```python
from build123d import *

# Parameters (mm, degrees)
SKETCH1_W                            = 127
SKETCH1_H                            = 50.8
BOSS_EXTRUDE1_DEPTH                  = 25.4
SKETCH2_R                            = 4.5085
CUT_EXTRUDE1_DEPTH                   = 73.955945611
SKETCH3_W                            = 19.05
SKETCH3_H                            = 1.5875
CUT_EXTRUDE2_DEPTH                   = 73.955945611
SKETCH4_W                            = 12.7
SKETCH4_H                            = 14.605
CUT_EXTRUDE3_DEPTH                   = 73.955945611
F_11_64_0_17188_DIAMETER_HOLE1_D     = 4.365752
F_11_64_0_17188_DIAMETER_HOLE1_DEPTH = 25.4
F_11_64_0_17188_DIAMETER_HOLE1_TIP   = 1.311604225
FILLET3_R                            = 2.54
F_11_64_0_17188_DIAMETER_HOLE2_D     = 4.365752
F_11_64_0_17188_DIAMETER_HOLE2_DEPTH = 25.4
F_11_64_0_17188_DIAMETER_HOLE2_TIP   = 1.311604225
SKETCH9_W                            = 44.45
SKETCH9_H                            = 6.35
CUT_EXTRUDE4_DEPTH                   = 73.955945611


with BuildPart() as part:
    # Sketch1 → Boss-Extrude1 (new body)
    with BuildSketch(Plane(origin=(0, 0, 0), x_dir=(1, 0, 0), z_dir=(0, 1, 0))):
        Rectangle(SKETCH1_W, SKETCH1_H)
    extrude(amount=BOSS_EXTRUDE1_DEPTH)

    # Sketch2 → Cut-Extrude1 (cut, through all)
    with BuildSketch(Plane(origin=(0, 25.4, 0), x_dir=(1, 0, 0), z_dir=(0, 1, 0))):
        with Locations(Location((-44.45, 0, 0), (0, 0, 270))):
            Circle(SKETCH2_R)
        with Locations(Location((44.45, 0, 0), (0, 0, 270))):
            Circle(SKETCH2_R)
    extrude(amount=-CUT_EXTRUDE1_DEPTH, mode=Mode.SUBTRACT)

    # Sketch3 → Cut-Extrude2 (cut, through all)
    with BuildSketch(Plane(origin=(0, 25.4, 0), x_dir=(1, 0, 0), z_dir=(0, 1, 0))):
        with Locations((-53.975, 0)):
            Rectangle(SKETCH3_W, SKETCH3_H)
        with Locations((53.975, 0)):
            Rectangle(SKETCH3_W, SKETCH3_H)
    extrude(amount=-CUT_EXTRUDE2_DEPTH, mode=Mode.SUBTRACT)

    # Sketch4 → Cut-Extrude3 (cut, through all)
    with BuildSketch(Plane(origin=(0, 25.4, 0), x_dir=(1, 0, 0), z_dir=(0, 1, 0))):
        with Locations((-57.15, -18.0975)):
            Rectangle(SKETCH4_W, SKETCH4_H)
        with Locations((-57.15, 18.0975)):
            Rectangle(SKETCH4_W, SKETCH4_H)
        with Locations((57.15, 18.0975)):
            Rectangle(SKETCH4_W, SKETCH4_H)
        with Locations((57.15, -18.0975)):
            Rectangle(SKETCH4_W, SKETCH4_H)
    extrude(amount=-CUT_EXTRUDE3_DEPTH, mode=Mode.SUBTRACT)

    # 11/64 (0.17188) Diameter Hole1
    with Locations(Plane(origin=(-57.15, 20.32, 10.795), x_dir=(1, 0, 0), z_dir=(0, 0, 1))):
        with Locations((0, 0), (0, -15.24), (114.3, 0), (114.3, -15.24)):
            Hole(F_11_64_0_17188_DIAMETER_HOLE1_D / 2, depth=F_11_64_0_17188_DIAMETER_HOLE1_DEPTH)
            with Locations((0, 0, -(F_11_64_0_17188_DIAMETER_HOLE1_DEPTH + F_11_64_0_17188_DIAMETER_HOLE1_TIP / 2))):  # 118° drill point
                Cone(0, F_11_64_0_17188_DIAMETER_HOLE1_D / 2, F_11_64_0_17188_DIAMETER_HOLE1_TIP, mode=Mode.SUBTRACT)

    # Fillet3
    fillet3_edges = [part.edges().sort_by_distance(p)[0] for p in [
        (50.8, 12.7, 10.795),
        (-50.8, 12.7, 10.795),
        (-50.8, 12.7, -10.795),
        (50.8, 12.7, -10.795),
    ]]
    fillet(fillet3_edges, radius=FILLET3_R)

    # 11/64 (0.17188) Diameter Hole2
    with Locations(Plane(origin=(-44.45, 25.4, -19.05), x_dir=(0, 0, 1), z_dir=(0, 1, 0))):
        with Locations((0, 0), (38.1, 0), (38.1, 88.9), (0, 88.9)):
            Hole(F_11_64_0_17188_DIAMETER_HOLE2_D / 2, depth=F_11_64_0_17188_DIAMETER_HOLE2_DEPTH)
            with Locations((0, 0, -(F_11_64_0_17188_DIAMETER_HOLE2_DEPTH + F_11_64_0_17188_DIAMETER_HOLE2_TIP / 2))):  # 118° drill point
                Cone(0, F_11_64_0_17188_DIAMETER_HOLE2_D / 2, F_11_64_0_17188_DIAMETER_HOLE2_TIP, mode=Mode.SUBTRACT)

    # Sketch9 → Cut-Extrude4 (cut, through all)
    with BuildSketch(Plane(origin=(0, 25.4, 0), x_dir=(1, 0, 0), z_dir=(0, 1, 0))):
        with Locations((0, -22.225)):
            Rectangle(SKETCH9_W, SKETCH9_H)
        with Locations((0, 22.225)):
            Rectangle(SKETCH9_W, SKETCH9_H)
    extrude(amount=-CUT_EXTRUDE4_DEPTH, mode=Mode.SUBTRACT)


solid = part.part
```
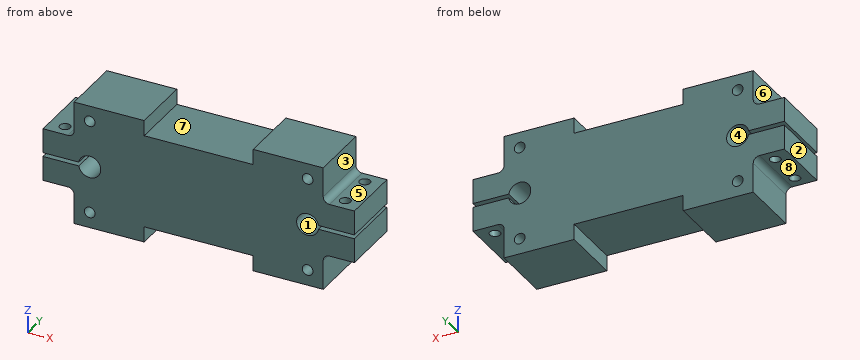
Could you check a few things on this model? Use its own coordinates, in mm. Face numbers are marked on the shaded views. A direction names the side the tool comes from. Round coordinates to 2 decimals unless told otherwise and drop trailing zeros. Write each loop counter-clockwise with the first axis right and the second up, starting at its lowest first coordinate (ties: lowest second). Pieces come first, ordered by that corner, then holes. Notation, with made-up numbers: M 18.25,23 L 77.25,23 A24 ccw 77.25,35 Z; hole C 49.5,-18 d3. An arc over 180 degrees is marked long. Write each question's results on one line, items separated by ' | '. Start each with the question number.
1. I need wall thicknesses on L1, parallel to Z at x = -44.45, y = 6.25; L2, parallel to Y at x = -57, z = -8; L3, parallel to Z at x = -43.5, y = 10. Which ranges of each line are inside material? Lowest first, please. Write a range as from..to.
2. Thinking about a two-plate mould opening in X: for the marked faces 1, 2, 3 and 4, which applies, +X half, -X half, draft (parallel to the pull), parting line (faces both ways), or undercut?
3. Imagine slicing it at A-A on x = -44.45. List the corners of the cut face in (y, z) for me, and give its area (3 significant figures).
4. I'm going to push flat-ended pins straight in: pin 1 Ø3 at (y, z) = (11, 22) entering from -X; pin 2 Ø1.9 at (y, z) = (13, 21) entering from +X; pin 3 Ø8 at (x, y) = (-56, 8.5) entering from +Z. Where does each tip first touch, or does it pass through?
5. Imagine slicing it at B-B on z = 7. List the corners of the cut face in (x, y) for me, and give its area (3 significant figures).
6. On a 3-axis mill with a long thin cutter (end or side, diameter ignored), from which of +Z, -Z, +X, -X, +Y, -Y can I reach the whole of each face in a straight line? I mean the marked faces 5, 6, 7 and 8. Say none if no direction works.
7. Imagine slicing it at C-C on x = 57.15. List the corners of the cut face in (y, z) for me (3 decimals).
8. Imagine slicing it at D-D on y = 20.32. Count the separate pieces of the cut face and the enclosed holes in it, and give its area (3 significant figures).
Result sheet:
1) L1: z = -25.4..-21.23, -16.87..-4.51, 4.51..16.87, 21.23..25.4 | L2: y = 0..2.9, 7.26..18.14, 22.5..25.4 | L3: z = -25.4..-21.02, -17.08..-4.41, 4.41..17.08, 21.02..25.4
2) face 1: undercut | face 2: -X half | face 3: +X half | face 4: undercut
3) outline: M 0,-25.4 L 25.4,-25.4 L 25.4,-21.23 L 0,-21.23 Z; M 0,-16.87 L 25.4,-16.87 L 25.4,-4.51 L 0,-4.51 Z; M 0,4.51 L 25.4,4.51 L 25.4,16.87 L 0,16.87 Z; M 0,21.23 L 25.4,21.23 L 25.4,25.4 L 0,25.4 Z | area: 840 mm^2
4) pin 1: stops at x = -50.8 | pin 2: stops at x = 50.8 | pin 3: stops at z = 11.18
5) outline: M -63.5,0 L 63.5,0 L 63.5,25.4 L -63.5,25.4 Z; hole C -57.15,5.08 d4.37; hole C -57.15,20.32 d4.37; hole C 57.15,5.08 d4.37; hole C 57.15,20.32 d4.37 | area: 3,170 mm^2
6) face 5: +Z, +X, +Y, -Y | face 6: +Z, -X, +Y, -Y | face 7: +Z, +Y, -Y | face 8: -Z, -X, +Y, -Y
7) outline: M 0,-10.795 L 2.897,-10.795 L 2.897,-0.794 L 0,-0.794 Z; M 0,0.794 L 2.897,0.794 L 2.897,10.795 L 0,10.795 Z; M 7.263,-10.795 L 18.137,-10.795 L 18.137,-0.794 L 7.263,-0.794 Z; M 7.263,0.794 L 18.137,0.794 L 18.137,10.795 L 7.263,10.795 Z; M 22.503,-10.795 L 25.4,-10.795 L 25.4,-0.794 L 22.503,-0.794 Z; M 22.503,0.794 L 25.4,0.794 L 25.4,10.795 L 22.503,10.795 Z
8) separate pieces: 5 | enclosed holes: 4 | area: 4,740 mm^2
